Autodesk Inventor part; units mm, degrees
ref_plane "YZ Plane" through (0, 0, 0) normal (1, 0, 0) x (0, 1, 0)
ref_plane "XZ Plane" through (0, 0, 0) normal (0, 1, 0) x (-1, 0, 0)
ref_plane "XY Plane" through (0, 0, 0) normal (0, 0, 1) x (1, 0, 0)
sketch "Sketch1" plane through (0, 0, 0) normal (0, 1, 0) x (-1, 0, 0)
  circle A0 centre (0.6883, 0.5378) radius 860
  point P0 (0, 0)
  dimension "d0" = 1720
extrude "Extrusion1" add sketch "Sketch1" along normal blind 2.54
sketch "Sketch2" plane through (-0.6883, 2.54, 0.5378) normal (0, 1, 0) x (1, 0, 0)
  circle A0 centre (0.6883, 0.5378) radius 45
  dimension "d7" = 90
extrude "Extrusion2" cut sketch "Sketch2" against normal blind 25.4
sketch "Sketch3" plane through (-0.6883, 2.54, 0.5378) normal (0, 1, 0) x (1, 0, 0)
  circle A0 centre (0, 0) radius 860
  line L0 (-893.9159, 16.958) -> (-826.0841, 16.958)
  line L1 (-826.0841, 16.958) -> (-826.0841, -16.958)
  line L2 (-826.0841, -16.958) -> (-893.9159, -16.958)
  line L3 (-893.9159, -16.958) -> (-893.9159, 16.958)
  line L4 (-860, 16.958) -> (-860, -16.958) construction
  line L5 (0, 0) -> (-860, 0) construction
extrude "Extrusion3" cut sketch "Sketch3" against normal blind 10 contours L0 L1 L2 A0 | A0 L2 L3 L0 picked at (-837.3832, 1.8843)
pattern_circular "Circular Pattern1" count 6 over 360 about axis through (0, 2.54, 0) along (0, -1, 0) of "Extrusion3"
properties part number "2f2surf" material "Glass"
For this review, take the finished solid that the model builds, in its own axes (mm). Round coordinates to 2 decimals unless told otherwise and drop trailing zeros. Write each loop counter-clockwise with the first axis right and the second up, starting at its lowest first coordinate (ties: lowest second). Pieces come first, ordered by that corner, then holes. Notation, with made-up numbers: M 1,65 L 60,65 A29 cw 60,86 Z; hole C 65,57 d7. An arc over 180 degrees is marked long. One line per item, written item: value. Start each with the question number.
(1) Insertion check: pin 1 (1.3 mm diameter, centred on y = 1.5, z = 1, fed in from +X). The pin has a flat end and moves straight along its axis. Give the tip position at first contact, or say it passes through.
(2) We need section C-C (z = -340.5). Give the boundary of the cut face in (x, y).
(3) We need section A-A (x = 0). Give the boundary of the cut face in (y, z), and give its area (3 significant figures).
(4) We need section B-B (y = 0.5). Give the boundary of the cut face in (x, z), and give its area (3 significant figures).
(5) We need section D-D (z = 557). Give the boundary of the cut face in (x, y), and give its area (3 significant figures).
(6) Wall thickness on line 1 (Z direction, x = 0, y = 0.9); line 2 (X direction, y = 1.85, z = 0); line 3 (Z direction, x = 80, y = 0.7): over which ranges is each line inside the solid? List them lowest first.
(7) The part is to be moulded in two halves that separate along X. For faces 1 (the cylindrical face through (6.516, 1.252, 860.508)), 2 (the cylindrical face through (-742.196, 1.252, 436.159)), 3 (the cylindrical face through (20.765, 1.288, 39.923)), say which applies: released by +X, released by -X, zero draft, split by the parting line, or undercut.
Result:
1. pin 1: x = 826.77
2. outline: M -790.18,0 L 788.8,0 L 788.8,2.54 L -790.18,2.54 Z
3. outline: M 0,-859.46 L 2.54,-859.46 L 2.54,-45 L 0,-45 Z; M 0,45 L 2.54,45 L 2.54,860.54 L 0,860.54 Z
3. area: 4,140 mm²
4. outline: M -860.52,-16.42 A860 ccw -445.01,-735.79 L -428.54,-707.26 L -399.17,-724.22 L -415.63,-752.74 A860 ccw 414.36,-752.68 L 398.23,-724.75 L 427.61,-707.8 L 443.73,-735.73 A860 ccw 859.12,-17.5 L 826.77,-17.5 L 826.77,16.42 L 859.17,16.42 A860 ccw 445.11,735.97 L 428.54,707.26 L 399.17,724.22 L 415.77,752.98 A860 ccw -415.16,754.07 L -398.23,724.75 L -427.61,707.8 L -444.55,737.14 A860 ccw -860.52,17.5 L -826.77,17.5 L -826.77,-16.42 Z; hole C 0,0 d90
4. area: 2,310,000 mm²
5. outline: M -656.39,0 L 655.02,0 L 655.02,2.54 L -656.39,2.54 Z
5. area: 3,330 mm²
6. line 1: -859.46 to -45, 45 to 860.54
6. line 2: -826.77 to -45, 45 to 826.77
6. line 3: -855.67 to 856.74
7. face 1: split by the parting line
7. face 2: released by -X
7. face 3: undercut
